```python
from build123d import *

# Parameters (mm, degrees)
SKETCH1_R           = 2
BOSS_EXTRUDE1_DEPTH = 6.35
CHAMFER1_SIZE       = 2.54
CUT_EXTRUDE1_DEPTH  = 4.7625
FILLET1_R           = 4
FILLET2_R           = 2


with BuildPart() as part:
    # Sketch1 → Boss-Extrude1 (new body)
    with BuildSketch(Plane(origin=(0, 0, 0), x_dir=(1, 0, 0), z_dir=(0, 1, 0))):
        with BuildLine():
            Line((-42.746, 11.684), (47.586884748, 11.684))
            Line((47.586884748, 11.684), (47.586884748, 17.78))
            ThreePointArc((47.586884748, 17.78), (31.011055518, 40.236232871), (5.073646026, 50.546))
            Line((5.073646026, 50.546), (-5.073646026, 50.546))
            ThreePointArc((-5.073646026, 50.546), (-26.552841725, 43.308043091), (-42.746, 27.448487827))
            Line((-42.746, 27.448487827), (-42.746, 11.684))
        make_face()
        with Locations((0, 17.78)):
            Circle(SKETCH1_R, mode=Mode.SUBTRACT)
        with Locations((0, 43.18)):
            Circle(SKETCH1_R, mode=Mode.SUBTRACT)
        with BuildLine():
            Line((47.586884748, 17.78), (47.586884748, 11.684))
            Line((47.586884748, 11.684), (49.243425186, 11.684))
            Line((49.243425186, 11.684), (49.243425186, 12.478985375))
            ThreePointArc((49.243425186, 12.478985375), (48.487652237, 15.15214772), (47.586884748, 17.78))
        make_face()
        with BuildLine():
            Line((-5.073646026, 50.546), (5.073646026, 50.546))
            ThreePointArc((5.073646026, 50.546), (2.539999948, 50.736460265), (-1.05e-07, 50.8))
            ThreePointArc((-1.05e-07, 50.8), (-2.540000052, 50.73646026), (-5.073646026, 50.546))
        make_face()
    extrude(amount=BOSS_EXTRUDE1_DEPTH)

    # Chamfer1
    chamfer1_edges = [part.edges().sort_by_distance(p)[0] for p in [
        (-2, 6.35, -17.78),
        (-2, 6.35, -43.18),
    ]]
    chamfer(chamfer1_edges, length=CHAMFER1_SIZE)

    # Sketch2 → Cut-Extrude1 (cut)
    with BuildSketch(Plane.XZ):
        with BuildLine():
            ThreePointArc((4.836612521, -48.974251761), (31.631563601, -37.700322816), (47.389212317, -13.2715))
            Line((47.389212317, -13.2715), (5.450452083, -13.2715))
            ThreePointArc((5.450452083, -13.2715), (3.766359845, -14.192688904), (3.633634696, -16.107666631))
            ThreePointArc((3.633634696, -16.107666631), (1e-09, -21.78), (-3.633634697, -16.107666633))
            ThreePointArc((-3.633634697, -16.107666633), (-3.766359842, -14.192688907), (-5.450452076, -13.2715))
            Line((-5.450452076, -13.2715), (-41.1585, -13.2715))
            Line((-41.1585, -13.2715), (-41.1585, -26.978658862))
            ThreePointArc((-41.1585, -26.978658862), (-25.491942293, -42.09549898), (-4.836612574, -48.974251756))
            ThreePointArc((-4.836612574, -48.974251756), (-2.876580864, -47.927421723), (-3.093368257, -45.715955999))
            ThreePointArc((-3.093368257, -45.715955999), (1e-09, -39.18), (3.093368255, -45.715956001))
            ThreePointArc((3.093368255, -45.715956001), (2.876580852, -47.927421701), (4.836612521, -48.974251761))
        make_face()
    extrude(amount=-CUT_EXTRUDE1_DEPTH, mode=Mode.SUBTRACT)

    # Fillet1
    fillet1_edges = [part.edges().sort_by_distance(p)[0] for p in [
        (47.389212317, 2.38125, -13.2715),
        (-41.1585, 2.38125, -13.2715),
        (-41.1585, 2.38125, -26.978658862),
    ]]
    fillet(fillet1_edges, radius=FILLET1_R)

    # Fillet2
    fillet2_edges = [part.edges().sort_by_distance(p)[0] for p in [
        (1e-09, 4.7625, -21.78),
        (1e-09, 4.7625, -39.18),
        (-2.876580864, 4.7625, -47.927421723),
        (2.876580852, 4.7625, -47.927421701),
        (29.335536204, 4.7625, -39.513244259),
        (3.766359845, 4.7625, -14.192688904),
        (-3.766359842, 4.7625, -14.192688907),
        (-21.304476038, 4.7625, -13.2715),
        (23.617003395, 4.7625, -13.2715),
        (-24.944627959, 4.7625, -42.422113246),
        (-41.1585, 4.7625, -21.514181912),
        (-39.986927125, 4.7625, -14.443072875),
        (-40.976209704, 4.7625, -26.950636255),
        (45.108619745, 4.7625, -15.048002194),
    ]]
    fillet(fillet2_edges, radius=FILLET2_R)


solid = part.part
```
Verification items for the finished model (mm, model axes). A direction names the side the tool comes from. Round coordinates to 2 decimals unless told otherwise and drop trailing zeros.
1. Scan lines: L1, parallel to X at y = 2.35, z = -17.78; L2, parallel to X at y = 1.4, z = -43.18; L3, parallel to X at y = 1, z = -14. Record each from-to range of solid material in increasing order.
2. Access from +Z, -Z, +X, -X, +Y, -Y to the whole of each face (thin tool, end or side, straight path). Record for faces 1 (the cylindrical face through (-0.26, 1.878, -19.763)), 2 (the cylindrical face through (-3.75, 1.36, -14.22)).
3. Gauge pin test, flat ends, axial feed: P1, Ø2, axis at x = -21.5, y = 2, coming from the -Z side; P2, Ø4.5, axis at x = 0, z = -43.18, coming from the +Y side; P3, Ø0.8, axis at x = 15.5, y = 2, coming from the -Z side. Record the tip position at first contact, or that the pin passes through.
4. Draft check along Z on faces 3 (the flat face through (3, 3, -11.684)), 4 (the flat face through (0, 0, -21)), 5 (the cylindrical face through (-40.018, 1.401, -14.474)). Enter one of: +Z half, -Z half, draft (parallel to the pull), parting line (faces both ways), or undercut.
5. Section check A-A on x = -1. State how many separate pieces and enclosed holes the cut face has, plus the area to 3 significant figures.
Answer:
1. L1: x = -42.75 to -41.16, -4 to -2, 2 to 4, 45.75 to 47.59
1. L2: x = -26.76 to -23.61, -4 to -2, 2 to 4, 23.61 to 26.76
1. L3: x = -42.75 to -39.46, -3.91 to 3.91, 44.09 to 48.83
2. face 1: +Y, -Y
2. face 2: -Y
3. P1: stops at z = -46.48
3. P2: stops at y = 4.06
3. P3: stops at z = -48.5
4. face 3: +Z half
4. face 4: draft
4. face 5: undercut
5. separate pieces: 3
5. enclosed holes: 0
5. area: 108 mm2
